from build123d import *

# Parameters (mm, degrees)
BOSS_EXTRUDE1_DEPTH = 31.75
CHAMFER1_SIZE       = 3.302
CUT_EXTRUDE1_REACH  = 67.596
SKETCH2_R           = 3.429
CUT_EXTRUDE2_REACH  = 70.999
SKETCH3_R           = 3.429
CHAMFER2_SIZE       = 0.762


with BuildPart() as part:
    # Sketch1 → Boss-Extrude1 (new body, symmetric)
    with BuildSketch(Plane.XY):
        with BuildLine():
            Line((0, 2.54), (0, 42.264401363))
            ThreePointArc((0, 42.264401363), (-0.340295474, 43.534401363), (-1.27, 44.464105889))
            Line((-1.27, 44.464105889), (-23.24261314, 57.15))
            Line((-23.24261314, 57.15), (-20.06761314, 62.649261314))
            Line((-20.06761314, 62.649261314), (34.925, 30.899261314))
            Line((34.925, 30.899261314), (31.75, 25.4))
            Line((31.75, 25.4), (10.16, 37.864992312))
            ThreePointArc((10.16, 37.864992312), (7.62, 37.864992312), (6.35, 35.665287786))
            Line((6.35, 35.665287786), (6.35, 2.54))
            ThreePointArc((6.35, 2.54), (7.093948776, 0.743948776), (8.89, 0))
            Line((8.89, 0), (44.45, 0))
            Line((44.45, 0), (44.45, -6.35))
            Line((44.45, -6.35), (-31.75, -6.35))
            Line((-31.75, -6.35), (-31.75, 0))
            Line((-31.75, 0), (-2.54, 0))
            ThreePointArc((-2.54, 0), (-0.743948776, 0.743948776), (0, 2.54))
        make_face()
    extrude(amount=BOSS_EXTRUDE1_DEPTH, both=True)

    # Chamfer1
    chamfer1_edges = [part.edges().sort_by_distance(p)[0] for p in [
        (33.3375, 28.149630657, -31.75),
        (44.45, -3.175, -31.75),
        (-31.75, -3.175, -31.75),
        (-21.65511314, 59.899630657, -31.75),
        (-31.75, -3.175, 31.75),
        (44.45, -3.175, 31.75),
        (-21.65511314, 59.899630657, 31.75),
        (33.3375, 28.149630657, 31.75),
    ]]
    chamfer(chamfer1_edges, length=CHAMFER1_SIZE)

    # Sketch2 → Cut-Extrude1 (cut, up to next)
    with BuildSketch(Plane(origin=(22.111022628, 38.297414599, 0), x_dir=(0.866025404, -0.5, 0), z_dir=(0.5, 0.866025404, 0)), mode=Mode.PRIVATE) as cut_extrude1_sk1:
        with Locations((-36.00369343, 19.05)):
            Circle(SKETCH2_R)
    cut_extrude1_tool1 = extrude(cut_extrude1_sk1.sketch, amount=-CUT_EXTRUDE1_REACH, mode=Mode.PRIVATE) & part.part
    add(cut_extrude1_tool1.solids().sort_by_distance((-9.069091, 56.299261, -19.05))[0], mode=Mode.SUBTRACT)
    # Sketch2 → Cut-Extrude1 (cut, up to next)
    with BuildSketch(Plane(origin=(22.111022628, 38.297414599, 0), x_dir=(0.866025404, -0.5, 0), z_dir=(0.5, 0.866025404, 0)), mode=Mode.PRIVATE) as cut_extrude1_sk2:
        with Locations((2.09630657, 19.05)):
            Circle(SKETCH2_R)
    cut_extrude1_tool2 = extrude(cut_extrude1_sk2.sketch, amount=-CUT_EXTRUDE1_REACH, mode=Mode.PRIVATE) & part.part
    add(cut_extrude1_tool2.solids().sort_by_distance((23.926477, 37.249261, -19.05))[0], mode=Mode.SUBTRACT)
    # Sketch2 → Cut-Extrude1 (cut, up to next)
    with BuildSketch(Plane(origin=(22.111022628, 38.297414599, 0), x_dir=(0.866025404, -0.5, 0), z_dir=(0.5, 0.866025404, 0)), mode=Mode.PRIVATE) as cut_extrude1_sk3:
        with Locations((-36.00369343, -19.05)):
            Circle(SKETCH2_R)
    cut_extrude1_tool3 = extrude(cut_extrude1_sk3.sketch, amount=-CUT_EXTRUDE1_REACH, mode=Mode.PRIVATE) & part.part
    add(cut_extrude1_tool3.solids().sort_by_distance((-9.069091, 56.299261, 19.05))[0], mode=Mode.SUBTRACT)
    # Sketch2 → Cut-Extrude1 (cut, up to next)
    with BuildSketch(Plane(origin=(22.111022628, 38.297414599, 0), x_dir=(0.866025404, -0.5, 0), z_dir=(0.5, 0.866025404, 0)), mode=Mode.PRIVATE) as cut_extrude1_sk4:
        with Locations((2.09630657, -19.05)):
            Circle(SKETCH2_R)
    cut_extrude1_tool4 = extrude(cut_extrude1_sk4.sketch, amount=-CUT_EXTRUDE1_REACH, mode=Mode.PRIVATE) & part.part
    add(cut_extrude1_tool4.solids().sort_by_distance((23.926477, 37.249261, 19.05))[0], mode=Mode.SUBTRACT)

    # Sketch3 → Cut-Extrude2 (cut, up to next)
    with BuildSketch(Plane.XZ.offset(6.35), mode=Mode.PRIVATE) as cut_extrude2_sk1:
        with Locations((-23.8125, 23.8125)):
            Circle(SKETCH3_R)
    cut_extrude2_tool1 = extrude(cut_extrude2_sk1.sketch, amount=-CUT_EXTRUDE2_REACH, mode=Mode.PRIVATE) & part.part
    add(cut_extrude2_tool1.solids().sort_by_distance((-23.8125, -6.35, 23.8125))[0], mode=Mode.SUBTRACT)
    # Sketch3 → Cut-Extrude2 (cut, up to next)
    with BuildSketch(Plane.XZ.offset(6.35), mode=Mode.PRIVATE) as cut_extrude2_sk2:
        with Locations((36.5125, 23.8125)):
            Circle(SKETCH3_R)
    cut_extrude2_tool2 = extrude(cut_extrude2_sk2.sketch, amount=-CUT_EXTRUDE2_REACH, mode=Mode.PRIVATE) & part.part
    add(cut_extrude2_tool2.solids().sort_by_distance((36.5125, -6.35, 23.8125))[0], mode=Mode.SUBTRACT)
    # Sketch3 → Cut-Extrude2 (cut, up to next)
    with BuildSketch(Plane.XZ.offset(6.35), mode=Mode.PRIVATE) as cut_extrude2_sk3:
        with Locations((-23.8125, -23.8125)):
            Circle(SKETCH3_R)
    cut_extrude2_tool3 = extrude(cut_extrude2_sk3.sketch, amount=-CUT_EXTRUDE2_REACH, mode=Mode.PRIVATE) & part.part
    add(cut_extrude2_tool3.solids().sort_by_distance((-23.8125, -6.35, -23.8125))[0], mode=Mode.SUBTRACT)
    # Sketch3 → Cut-Extrude2 (cut, up to next)
    with BuildSketch(Plane.XZ.offset(6.35), mode=Mode.PRIVATE) as cut_extrude2_sk4:
        with Locations((36.5125, -23.8125)):
            Circle(SKETCH3_R)
    cut_extrude2_tool4 = extrude(cut_extrude2_sk4.sketch, amount=-CUT_EXTRUDE2_REACH, mode=Mode.PRIVATE) & part.part
    add(cut_extrude2_tool4.solids().sort_by_distance((36.5125, -6.35, -23.8125))[0], mode=Mode.SUBTRACT)

    # Chamfer2
    chamfer2_edges = [part.edges().sort_by_distance(p)[0] for p in [
        (17.781876262, 33.4645, -19.05),
        (20.956876262, 38.963761314, -19.05),
        (-12.038691622, 58.013761314, 19.05),
        (-15.213691622, 52.5145, 19.05),
        (17.781876262, 33.4645, 19.05),
        (20.956876262, 38.963761314, 19.05),
        (-12.038691622, 58.013761314, -19.05),
        (-15.213691622, 52.5145, -19.05),
        (33.0835, -6.35, 23.8125),
        (33.0835, 0, 23.8125),
        (-27.2415, -6.35, -23.8125),
        (-27.2415, 0, -23.8125),
        (33.0835, -6.35, -23.8125),
        (33.0835, 0, -23.8125),
        (-27.2415, -6.35, 23.8125),
        (-27.2415, 0, 23.8125),
    ]]
    chamfer(chamfer2_edges, length=CHAMFER2_SIZE)


solid = part.part
Geometry check sheet. Reference: the model listing, model coordinates, mm. A direction names the side the tool comes from. Round coordinates to 2 decimals unless told otherwise and drop trailing zeros. Loops run counter-clockwise (first coordinate to the right, second up) from the corner with the lowest first, then second, coordinate; pieces in that order, holes last. Notation, with made-up numbers: (4.25, -39) - (41.25, -39) arc R15 ccw to (41.25, -16) - close; hole circle Ø6 at (76, -25). An arc over 180 degrees is marked (long way). One line per question, with ' | ' between items. Start each with the question number.
1. Cross-section at A-A on x = 13.5. Record the cut outline in (y, z), then the cut area to 3 significant figures.
2. Cross-section at B-B on z = -12.5. Record the cut outline in (x, y) (3 decimals), then the cut area to 3 significant figures.
3. Cross-section at C-C on y = 12.5. Record the cut outline in (x, z), then the cut area to 3 significant figures.
4. Cross-section at D-D on x = -22. State how many separate pieces and enclosed holes the cut face has, then the cut area to 3 significant figures.
5. Tool access check on faces 4 (the face through (26, 0, 0)), 5 (the face through (6.35, 19, 0)), 6 (the face through (31.91, 29.025, -30.122)), 7 (the face through (36.066, -3.209, -20.413)), 8 (the face through (-0.764, 0.724, 0.444)). Record the directions out of +Z, -Z, +X, -X, +Y, -Y that give a thin tool (end or side, any length) a straight path to the whole face; none if there is none.
6. Draft check along X on faces 1 (the face through (-24.259, -3.209, 27.212)), 2 (the face through (-12.102, 50.718, 0.444)), 3 (the face through (33.36, 28.19, 0.4)). Enter one of: released by +X, released by -X, zero draft, split by the parting line, or undercut.
7. Depth check by flat-ended pin: pin 1 (5 mm diameter, centred on x = -8, z = -10, fed in from +Y); pin 2 (6 mm diameter, centred on y = 10, z = 21, fed in from +X); pin 3 (10.5 mm diameter, centred on x = 23.5, z = -11, fed in from +Y). Enter the tip coordinate at first touch or a pass-through.
8. Scan lines: line 1 (Z direction, x = 26, y = 35); line 2 (X direction, y = 23, z = -1.5); line 3 (Y direction, x = 7, z = -28). Record each from-to range of solid material in increasing order. Write a range as [from, to].
Taken from the geometry:
1) outline: (-6.35, -31.75) - (0, -31.75) - (0, 31.75) - (-6.35, 31.75) - close; (35.94, -31.75) - (43.27, -31.75) - (43.27, 31.75) - (35.94, 31.75) - close | area: 869 mm²
2) outline: (-31.75, -6.35) - (44.45, -6.35) - (44.45, 0) - (8.89, 0) arc R2.54 cw to (6.35, 2.54) - (6.35, 35.665) arc R2.54 cw to (10.16, 37.865) - (31.75, 25.4) - (34.925, 30.899) - (-20.068, 62.649) - (-23.243, 57.15) - (-1.27, 44.464) arc R2.54 cw to (0, 42.264) - (0, 2.54) arc R2.54 cw to (-2.54, 0) - (-31.75, 0) - close | area: 1,160 mm²
3) outline: (0, -31.75) - (6.35, -31.75) - (6.35, 31.75) - (0, 31.75) - close | area: 403 mm²
4) separate pieces: 4 | enclosed holes: 0 | area: 494 mm²
5) face 4: +Z, -Z, +X | face 5: +Z, -Z | face 6: -Z, +X | face 7: -Y | face 8: +Z, -Z, -X
6) face 1: undercut | face 2: released by -X | face 3: released by +X
7) pin 1: y = 57.13 | pin 2: x = 6.35 | pin 3: y = 40.53
8) line 1: [-31.75, -20.85], [-17.25, 17.25], [20.85, 31.75] | line 2: [0, 6.35] | line 3: [-6.35, 0.84], [37.36, 47.02]
